Can you work these out from the model? Positions are in its coordinate system, mm. Round coordinates to 2 decimals unless told otherwise and drop trailing zeros. Order: outer loops, then holes, each group sorted by start corner. A loop starts at its lowest first (then second) coordinate and runs counter-clockwise, first axis right, second up.
Autodesk Inventor part; units mm, degrees
ref_plane "YZ Plane" through (0, 0, 0) normal (1, 0, 0) x (0, 1, 0)
ref_plane "XZ Plane" through (0, 0, 0) normal (0, 1, 0) x (-1, 0, 0)
ref_plane "XY Plane" through (0, 0, 0) normal (0, 0, 1) x (1, 0, 0)
sketch "Sketch2" plane through (0, 0, 0) normal (1, 0, 0) x (0, 1, 0)
  line L0 (0, 0) -> (-40, 0)
  line L1 (-40, 0) -> (-40, -205)
  line L2 (-40, -205) -> (0, -205)
  line L3 (0, -205) -> (0, 0)
  line L4 (0, 0) -> (0, -5)
  line L5 (0, -5) -> (-5, -5)
  circle A0 centre (-5, -5) radius 1.5
  line L6 (-5, -5) -> (-5, -15)
  circle A1 centre (-5, -15) radius 1.5
  line L7 (0, -102.5) -> (-40, -102.5)
  circle A2 centre (-5, -200) radius 1.5
  circle A3 centre (-5, -190) radius 1.5
  line L8 (-40, 0) -> (-40, -10)
  line L9 (-40, -10) -> (-30, -10)
  line L10 (-30, -10) -> (-20, -10)
  circle A4 centre (-20, -10) radius 1.5
  circle A5 centre (-30, -10) radius 1.5
  circle A6 centre (-20, -195) radius 1.5
  circle A7 centre (-30, -195) radius 1.5
  dimension "d11" = 40
  dimension "d12" = 205
  dimension "d13" = 5
  dimension "d14" = 5
  dimension "d15" = 3
  dimension "d16" = 10
  dimension "d17" = 3
  dimension "d18" = 10
  dimension "d19" = 10
  dimension "d20" = 10
  dimension "d21" = 3
  dimension "d22" = 3
extrude "Extrusion3" add sketch "Sketch2" along normal blind 2
sketch "Sketch3" plane through (2, 0, 0) normal (1, 0, 0) x (0, 0, -1)
  line L0 (205, -40) -> (205, 0)
  line L1 (0, 0) -> (205, 0)
  line L2 (205, 0) -> (205, -15)
  line L3 (205, -15) -> (0, -15)
  line L4 (0, -15) -> (0, 0)
  dimension "d25" = 15
extrude "Extrusion4" cut sketch "Sketch3" against normal blind 2
sketch "Sketch4" plane through (2, 0, 0) normal (1, 0, 0) x (0, 0, -1)
  line L0 (0, -15) -> (0, -40)
  line L1 (0, -15) -> (25, -15)
  line L2 (0, -15) -> (205, -15)
  line L3 (25, -15) -> (25, -25)
  line L4 (25, -25) -> (0, -25)
  line L5 (205, -40) -> (205, -15)
  line L6 (205, -15) -> (180, -15)
  line L7 (180, -15) -> (180, -25)
  line L8 (180, -25) -> (205, -25)
  line L9 (205, -25) -> (205, -15)
  point P0 (0, 0)
  dimension "d28" = 25
  dimension "d29" = 10
  dimension "d30" = 25
extrude "Extrusion5" cut sketch "Sketch4" against normal blind 2
properties part number "plateHolder"
(1) I want a section at B-B, the plane y = -17. List the corners of the cut face in (x, z) for me.
(2) I want a section at A-A, the plane x = 1.6. List the corners of the cut face in (y, z) for me.
(3) I want a section at C-C, the plane z = -190.5. List the corners of the cut face in (x, y) for me.
(4) Please list where these lines run through material, in increasing order: probe 1 along Z at (x, y) = (1, -30); probe 2 along Y at (x, z) = (0.75, -195); probe 3 along Z at (x, y) = (1.7, -20.5).
(5) I'm going to push flat-ended pins straight in: pin 1 Ø1 at (x, y) = (0.5, -19) entering from +Z; pin 2 Ø0.6 at (x, z) = (1, -12.5) entering from +Y. Where does each tip first touch, or does it pass through?
Ans:
1. outline: (0, -180) - (2, -180) - (2, -25) - (0, -25) - close
2. outline: (-40, -205) - (-25, -205) - (-25, -180) - (-15, -180) - (-15, -25) - (-25, -25) - (-25, 0) - (-40, 0) - close; hole circle Ø3 at (-30, -195); hole circle Ø3 at (-30, -10)
3. outline: (0, -40) - (2, -40) - (2, -25) - (0, -25) - close
4. probe 1: z = -205 to -196.5, -193.5 to -11.5, -8.5 to 0
4. probe 2: y = -40 to -31.5, -28.5 to -25
4. probe 3: z = -180 to -25
5. pin 1: stops at z = -25
5. pin 2: stops at y = -25
